The listing builds one solid part. Answer for the finished solid, in the listing's coordinates (mm). Give positions to 0.01 mm unless a question says otherwise; leave off trailing zeros. Loops run counter-clockwise (first coordinate to the right, second up) from the corner with the lowest first, then second, coordinate; pieces in that order, holes last. Notation, with made-up numbers: (11.5, 2) - (69.5, 2) arc R10 cw to (69.5, 17) - close; hole circle Ø8 at (56, -30.75). An arc over 180 degrees is marked (long way). Answer as CSV lines item,"result". Start each with the question number.
1) A cutting plane is placed at A-A (x = 1.5). Determine the outline of the cut face in (y, z).
2) Find the intervals of material crossed by line 1 along Y through (x, z) = (-15.5, 2.25); line 2 along X through (y, z) = (0.7, -34); line 3 along Z through (x, y) = (-16.5, 5.5), in increasing order.
3) A cutting plane is placed at B-B (y = 3.5). Determine the outline of the cut face in (x, z), and give its area (3 significant figures).
4) Flat-ended cylindrical pins translate along their axes: pin 1 (2 mm diameter, centred on y = 3.5, z = 18.5, fed in from -X); pin 2 (1.3 mm diameter, centred on y = 0.5, z = -33.5, fed in from -X); pin 3 (12 mm diameter, centred on x = -14.5, z = 30.5, fed in from +Y); pin 4 (1.5 mm diameter, centred on x = -12.5, y = 2.5, fed in from +Z). Find the tip coordinate at first contact, or state that the pin passes through.
5) A cutting plane is placed at D-D (z = 23). Determine the outline of the cut face in (x, y).
6) A cutting plane is placed at C-C (z = -34). Determine the outline of the cut face in (x, y), and give its area (3 significant figures).
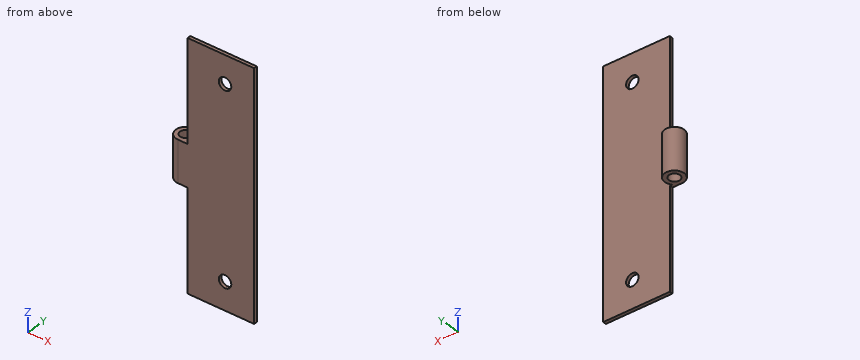
```python
from build123d import *

# Parameters (mm, degrees)
SKETCH1_W           = 24
SKETCH1_H           = 88
BOSS_EXTRUDE1_DEPTH = 1.2
SKETCH2_R           = 2
BOSS_EXTRUDE2_DEPTH = 7.5
SKETCH4_R           = 2.25
CUT_EXTRUDE2_DEPTH  = 49.276702456


with BuildPart() as part:
    # Sketch1 → Boss-Extrude1 (new body)
    with BuildSketch(Plane(origin=(0, 0, 0), x_dir=(1, 0, 0), z_dir=(0, 1, 0))):
        Rectangle(SKETCH1_W, SKETCH1_H)
    extrude(amount=BOSS_EXTRUDE1_DEPTH)

    # Sketch2 → Boss-Extrude2 (add, symmetric)
    with BuildSketch(Plane.XY):
        with BuildLine():
            Line((-12, 0), (-15.5, 0))
            ThreePointArc((-15.5, 0), (-16.949137675, 6.685906464), (-12.861818808, 1.2))
            Line((-12.861818808, 1.2), (-12, 1.2))
            Line((-12, 1.2), (-12, 0))
        make_face()
        with Locations((-15.5, 3.5)):
            Circle(SKETCH2_R, mode=Mode.SUBTRACT)
    extrude(amount=BOSS_EXTRUDE2_DEPTH, both=True)

    # Sketch4 → Cut-Extrude2 (cut, through all)
    with BuildSketch(Plane(origin=(0, 1.2, 0), x_dir=(1, 0, 0), z_dir=(0, 1, 0))):
        with Locations(Location((1.5, 34, 0), (0, 0, 270))):
            Circle(SKETCH4_R)
        with Locations(Location((1.5, -34, 0), (0, 0, 90))):
            Circle(SKETCH4_R)
    extrude(amount=-CUT_EXTRUDE2_DEPTH, mode=Mode.SUBTRACT)


solid = part.part
```
Ans:
1,outline,"(0, -44) - (1.2, -44) - (1.2, -36.25) - (0, -36.25) - close; (0, -31.75) - (1.2, -31.75) - (1.2, 31.75) - (0, 31.75) - close; (0, 36.25) - (1.2, 36.25) - (1.2, 44) - (0, 44) - close"
2,line 1,"0 to 1.5, 5.5 to 7"
2,line 2,"-12 to -0.75, 3.75 to 12"
2,line 3,"-7.5 to 7.5"
3,outline,"(-19, -7.5) - (-17.5, -7.5) - (-17.5, 7.5) - (-19, 7.5) - close; (-13.5, -7.5) - (-12, -7.5) - (-12, 7.5) - (-13.5, 7.5) - close"
3,area,"45.0 mm2"
4,pin 1,"through"
4,pin 2,"x = -12"
4,pin 3,"y = 1.2"
4,pin 4,"z = 7.5"
5,outline,"(-12, 0) - (12, 0) - (12, 1.2) - (-12, 1.2) - close"
6,outline,"(-12, 0) - (-0.75, 0) - (-0.75, 1.2) - (-12, 1.2) - close; (3.75, 0) - (12, 0) - (12, 1.2) - (3.75, 1.2) - close"
6,area,"23.4 mm2"
